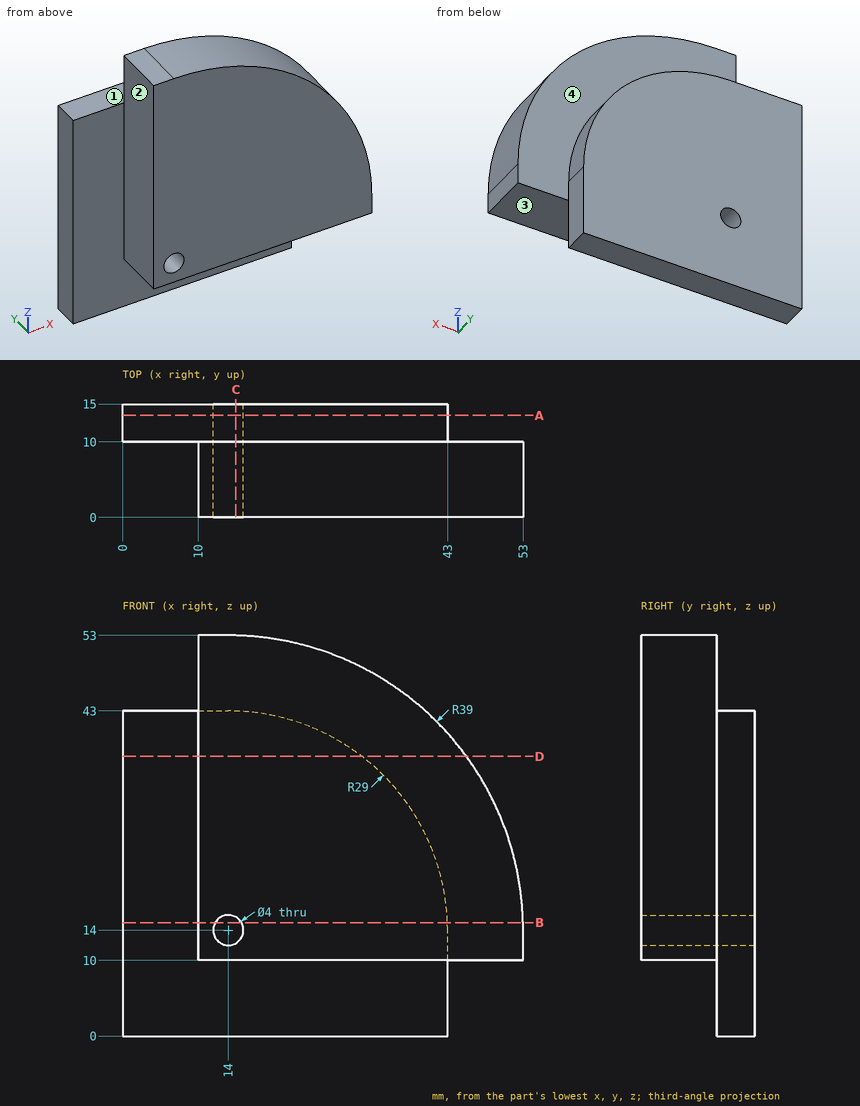
Drawing for the job (mm, zero at the part's lowest x, y, z). A direction names the side the tool comes from. Round coordinates to 2 decimals unless told otherwise and drop trailing zeros. Order: outer loops, then holes, each group sorted by start corner. A loop starts at its lowest first (then second) coordinate and runs counter-clockwise, first axis right, second up.
Item 1: Saw through at C-C on x = 15. Write the cut outline in (y, z).
Item 2: Pin check, flat tips, straight feed: pin 1 (2 mm diameter, centred on x = 11, y = 11.5, fed in from -Z); pin 2 (8 mm diameter, centred on y = 4, z = 36.5, fed in from -X); pin 3 (4 mm diameter, centred on x = 10, y = 13, fed in from +Z); pin 4 (12 mm diameter, centred on x = 46, z = 35, fed in from +Y). Stop position of each tip, or through.
Item 3: Probe line 1 along Z through (x, y) = (14, 8); line 2 along Z through (x, y) = (14, 10.25); line 3 along Y through (x, z) = (17.5, 8). List the from-to ranges inside material, lowest first.
Item 4: Saw through at B-B on z = 15. Write the cut outline in (x, y), then the cut area to 3 significant figures.
Item 5: Saw through at A-A on y = 13.5. Write the cut outline in (x, z), then the cut area to 3 significant figures.
Item 6: Saw through at D-D on z = 37. Write the cut outline in (x, y), then the cut area to 3 significant figures.
Item 7: Tool access for the marked faces 1, 2, 3 and 4: list every direction of +Z, -Z, +X, -X, +Y, -Y with a clear straight run to the whole face (end or side of a thin tool).
Reported:
1. outline: (0, 10) - (10, 10) - (10, 0) - (15, 0) - (15, 12.27) - (0, 12.27) - close; (0, 15.73) - (15, 15.73) - (15, 42.98) - (10, 42.98) - (10, 52.99) - (0, 52.99) - close
2. pin 1: stops at z = 0
2. pin 2: stops at x = 10
2. pin 3: stops at z = 43
2. pin 4: stops at y = 10
3. line 1: z = 10 to 12, 16 to 53
3. line 2: z = 0 to 12, 16 to 43
3. line 3: y = 10 to 15
4. outline: (0, 10) - (10, 10) - (10, 0) - (12.27, 0) - (12.27, 15) - (0, 15) - close; (15.73, 0) - (52.99, 0) - (52.99, 10) - (42.98, 10) - (42.98, 15) - (15.73, 15) - close
4. area: 593 mm2
5. outline: (0, 0) - (43, 0) - (43, 14) arc R29 ccw to (14, 43) - (0, 43) - close; hole circle Ø4 at (14, 14)
5. area: 1,660 mm2
6. outline: (0, 10) - (10, 10) - (10, 0) - (45.5, 0) - (45.5, 10) - (31.66, 10) - (31.66, 15) - (0, 15) - close
6. area: 513 mm2
7. face 1: +Z, +X, -X, +Y
7. face 2: +Z, -Z, -X, -Y
7. face 3: -Z, +X, -X, -Y
7. face 4: +Z, +X, +Y
